The listing builds one solid part. Answer for the finished solid, in the listing's coordinates (mm). A direction names the side the tool comes from. Round coordinates to 2 decimals unless told otherwise and drop trailing zeros. Loops run counter-clockwise (first coordinate to the right, second up) from the corner with the lowest first, then second, coordinate; pieces in that order, holes last. Notation, with made-up numbers: M -30,13.5 L -13,13.5 A14 cw -13,22.5 Z; hole C 69.25,22 d7. An arc over 180 degrees is marked long. Put each result on its own line as item: value. Start each with the question number.
(1) Straight lines are drawn through the part: line 1 (Z direction, x = 0, y = 2); line 2 (Z direction, x = 0, y = -3.75); line 3 (Y direction, x = 4.5, z = -5.25). For each, find the intervals that lie inside material, in ascending order.
(2) Determine the mould class of faces 1 (the face through (-0.867, -4.437, -3.905)), 2 (the face through (0, 3, 7)), 3 (the face through (1.847, -1.547, 0.766)) for opening direction X: released by +X, released by -X, zero draft, split by the parting line, or undercut.
(3) Section C-C, the plane y = 2.5 is taken. Determine the outline of the cut face in (x, z), then the cut area to 3 significant figures.
(4) Section A-A, the plane x = 0 is taken. Determine the outline of the cut face in (y, z).
(5) Which of the six approach directions +Z, -Z, +X, -X, +Y, -Y give full straight-line access (tool end or side, diameter ignored) to faces 4 (the face through (-4, 0, -2)), 5 (the face through (6.09, 2.96, -3.45))?
(6) Flat-ended cylindrical pins translate along their axes: P1, Ø1, axis at y = 2, z = 2, coming from the +X side; P2, Ø1, axis at x = 2, y = -5.5, coming from the +Z side; P3, Ø5, axis at y = -7, z = -3, coming from the +X side. Find the tip coordinate at first contact, or state that the pin passes through.
(7) Section B-B, the plane y = -5.25 is taken. Determine the outline of the cut face in (x, z).
(8) Section D-D, the plane z = 4.75 is taken. Determine the outline of the cut face in (x, y).
```python
from build123d import *

# Parameters (mm, degrees)
BOSS_EXTRUDE1_DEPTH = 6
FILLET1_R           = 0.5
SKETCH2_R           = 4
BOSS_EXTRUDE2_DEPTH = 9
SKETCH4_R           = 2
CUT_EXTRUDE1_DEPTH  = 16
CHAMFER1_SIZE       = 0.3
SKETCH5_R           = 1.5
CUT_EXTRUDE2_DEPTH  = 8


with BuildPart() as part:
    # Sketch1 → Boss-Extrude1 (new body)
    with BuildSketch(Plane(origin=(0, 0, 0), x_dir=(1, 0, 0), z_dir=(0, 1, 0))):
        Polygon((8.082903769, 0), (4.041451884, 7), (-4.041451884, 7), (-8.082903769, 0), (-4.041451884, -7), (4.041451884, -7), align=None)
    extrude(amount=BOSS_EXTRUDE1_DEPTH)

    # Fillet1
    fillet1_edges = [part.edges().sort_by_distance(p)[0] for p in [
        (4.041451884, 3, 7),
        (-4.041451884, 3, 7),
        (-8.082903769, 3, 0),
        (-4.041451884, 3, -7),
        (4.041451884, 3, -7),
        (8.082903769, 3, 0),
    ]]
    fillet(fillet1_edges, radius=FILLET1_R)

    # Sketch2 → Boss-Extrude2 (add)
    with BuildSketch(Plane.XZ):
        Circle(SKETCH2_R)
    extrude(amount=BOSS_EXTRUDE2_DEPTH)

    # Sketch4 → Cut-Extrude1 (cut, through all)
    with BuildSketch(Plane(origin=(0, 6, 0), x_dir=(1, 0, 0), z_dir=(0, 1, 0))):
        Circle(SKETCH4_R)
    extrude(amount=-CUT_EXTRUDE1_DEPTH, mode=Mode.SUBTRACT)

    # Chamfer1
    chamfer1_edges = [part.edges().sort_by_distance(p)[0] for p in [
        (-2, 6, 0),
    ]]
    chamfer(chamfer1_edges, length=CHAMFER1_SIZE)

    # Sketch5 → Cut-Extrude2 (cut)
    with BuildSketch(Plane(origin=(-6.062177826, 0, -3.5), x_dir=(-0.5, 0, 0.866025404), z_dir=(-0.866025404, 0, -0.5))):
        with Locations((0, 3)):
            Circle(SKETCH5_R)
    extrude(amount=-CUT_EXTRUDE2_DEPTH, mode=Mode.SUBTRACT)


solid = part.part
```
Recorded:
1. line 1: z = -7 to -2, 2 to 7
1. line 2: z = -4 to -2, 2 to 4
1. line 3: y = 0 to 6
2. face 1: split by the parting line
2. face 2: zero draft
2. face 3: undercut
3. outline: M -7.94,-0.25 L -6.77,-2.28 L -1.93,0.52 A2 cw long -0.52,-1.93 L -5.36,-4.72 L -4.19,-6.75 A0.5 ccw -3.75,-7 L 3.75,-7 A0.5 ccw 4.19,-6.75 L 7.94,-0.25 A0.5 ccw 7.94,0.25 L 4.19,6.75 A0.5 ccw 3.75,7 L -3.75,7 A0.5 ccw -4.19,6.75 L -7.94,0.25 A0.5 ccw Z
3. area: 142 mm²
4. outline: M -9,-4 L 0,-4 L 0,-7 L 6,-7 L 6,-2.3 L 5.7,-2 L -9,-2 Z; M -9,2 L 5.7,2 L 6,2.3 L 6,7 L 0,7 L 0,4 L -9,4 Z
5. face 4: -Y
5. face 5: -Z, +X, +Y, -Y
6. P1: stops at x = 7.22
6. P2: stops at z = 3.71
6. P3: stops at x = 3.97
7. outline: C 0,0 d8; hole C 0,0 d4
8. outline: M -5.34,0 L 5.34,0 L 5.34,6 L -5.34,6 Z
